Design review of the part built by this model. Coordinates are the model's own, in mm. A direction names the side the tool comes from. Round coordinates to 2 decimals unless told otherwise and drop trailing zeros. Order: outer loops, then holes, each group sorted by start corner. A loop starts at its lowest first (then second) coordinate and runs counter-clockwise, first axis right, second up. Notation, with made-up numbers: (79.5, 47) - (83.5, 47) arc R23 ccw to (83.5, 83) - close; hole circle Ø7 at (42, 67.25). An arc over 180 degrees is marked (long way). Write item = value, one per line.
from build123d import *

# Parameters (mm, degrees)
SKETCH1_R                = 46.99
BULKHEAD_EXTRUSION_DEPTH = 12.7
SKETCH2_R                = 1.6383
SCREW_HOLE_DEPTH         = 12.7
CIRPATTERN1_COUNT        = 8


with BuildPart() as part:
    # Sketch1 → Bulkhead Extrusion (new body)
    with BuildSketch(Plane(origin=(0, 0, 0), x_dir=(1, 0, 0), z_dir=(0, 1, 0))):
        with Locations(Location((0, 0, 0), (0, 0, 270))):
            Circle(SKETCH1_R)
    extrude(amount=BULKHEAD_EXTRUSION_DEPTH)

    # Sketch2 → Screw Hole (cut)
    with BuildSketch(Plane.XY.offset(46.99)):
        with Locations((0, 6.35)):
            Circle(SKETCH2_R)
    screw_hole = extrude(amount=-SCREW_HOLE_DEPTH, mode=Mode.SUBTRACT)

    # CirPattern1: Screw Hole ×8 about axis
    cirpattern1_axis = Axis((0, 0, 0), (0, 1, 0))
    for i in range(1, CIRPATTERN1_COUNT):
        add(screw_hole.rotate(cirpattern1_axis, i * 360 / CIRPATTERN1_COUNT), mode=Mode.SUBTRACT)


solid = part.part
Item 1: The part is to be moulded in two halves that separate along Y. For faces 4 (the face through (1, 0, -1)), 5 (the face through (1, 12.7, -1)), 6 (the face through (34.29, 6, 0)), say which applies: +Y half, -Y half, draft (parallel to the pull), parting line (faces both ways), or undercut.
Data:
face_4 = -Y half
face_5 = +Y half
face_6 = undercut
Item 2: For line 1 along Y through (x, z) = (0, -43.5); line 2 along X through (y, z) = (5.5, 25.5); line 3 along X through (y, z) = (7.5, -41), list the stretches that pass through material, from the lowest coordinate up. Write a range as [from, to].
Data:
line_1 = [0, 4.71], [7.99, 12.7]
line_2 = [-39.47, -27.48], [-23.52, 23.52], [27.48, 39.47]
line_3 = [-22.96, -1.17], [1.17, 22.96]
Item 3: Take a section at A-A, the plane x = 0. State the section outline as (y, z) points, and give its area (3 significant figures).
Data:
outline = (0, -46.99) - (4.71, -46.99) - (4.71, -34.29) - (7.99, -34.29) - (7.99, -46.99) - (12.7, -46.99) - (12.7, 46.99) - (7.99, 46.99) - (7.99, 34.29) - (4.71, 34.29) - (4.71, 46.99) - (0, 46.99) - close
area = 1,110 mm2
Item 4: Insertion check: P1, Ø2.5, axis at x = 0, y = 6.35, coming from the +Z side; P2, Ø2.5, axis at y = 6.35, z = 0, coming from the +X side; P3, Ø5, axis at y = 8.5, z = 27, coming from the -X side. Each pin has a flat end and moves straight along its axis. Give the tip position at first contact, or say it passes through.
Data:
P1 = 34.29
P2 = 34.29
P3 = -40.1
Item 5: Take a section at D-D, the plane z = 38.5. State the section outline as (x, y) points, and give its area (3 significant figures).
Data:
outline = (-26.94, 0) - (26.94, 0) - (26.94, 12.7) - (-26.94, 12.7) - close; hole circle Ø3.28 at (0, 6.35)
area = 676 mm2
Item 6: For faces 1 (the face through (0.36, 4.75, -40.73)), 2 (the face through (0, 6, 34.29)), 3 (the face through (24.263, 6.373, -24.23)), list the 3-axis set-ups (+Z, -Z, +X, -X, +Y, -Y) from which the entire face can be reached by the end or side of a thin tool; tool diameter is ignored.
Data:
face_1 = -Z
face_2 = +Z
face_3 = none
Item 7: Take a section at B-B, the plane z = 0. State the section outline as (x, y) points, and give its area (3 significant figures).
Data:
outline = (-46.99, 0) - (46.99, 0) - (46.99, 4.71) - (34.29, 4.71) - (34.29, 7.99) - (46.99, 7.99) - (46.99, 12.7) - (-46.99, 12.7) - (-46.99, 7.99) - (-34.29, 7.99) - (-34.29, 4.71) - (-46.99, 4.71) - close
area = 1,110 mm2
